Check sheet for the drawn part. Datum: minimum x, y, z corner. Units: mm. Give positions to 0.01 mm unless a question says otherwise; leave off trailing zeros. Order: outer loops, then holes, each group sorted by start corner. A loop starts at its lowest first (then second) coordinate and runs counter-clockwise, first axis right, second up. Notation, with made-up numbers: M -12.75,12.5 L 0.25,12.5 A14 cw 0.25,26.5 Z; hole C 75,23.5 d2. An arc over 180 degrees is marked long. Answer as CSV lines item,"result". Start each with the question number.
Q1. Section check A-A, the plane y = 0.85. Record the boundary of the cut face in (x, z).
Q2. Thickness scan on line 1 (X direction, y = 0.75, z = 48); line 2 (Z direction, x = 23.5, y = 0.65); line 3 (X direction, y = 1.4, z = 7). Record the ranges inside material, lowest first.
Q3. Go/stop test with flat-tipped pins: pin 1 (0.8 mm diameter, centred on y = 1, z = 47, fed in from -X); pin 2 (0.8 mm diameter, centred on y = 1, z = 11.5, fed in from +X); pin 3 (4 mm diameter, centred on x = 17, z = 43.5, fed in from -Y). Record where each tip stops, or that it passes through.
Q4. Section check C-C, the plane x = 12. Record the boundary of the cut face in (y, z) (1 decimal).
Q5. Section check B-B, the plane z = 11.5. Record the boundary of the cut face in (x, y).
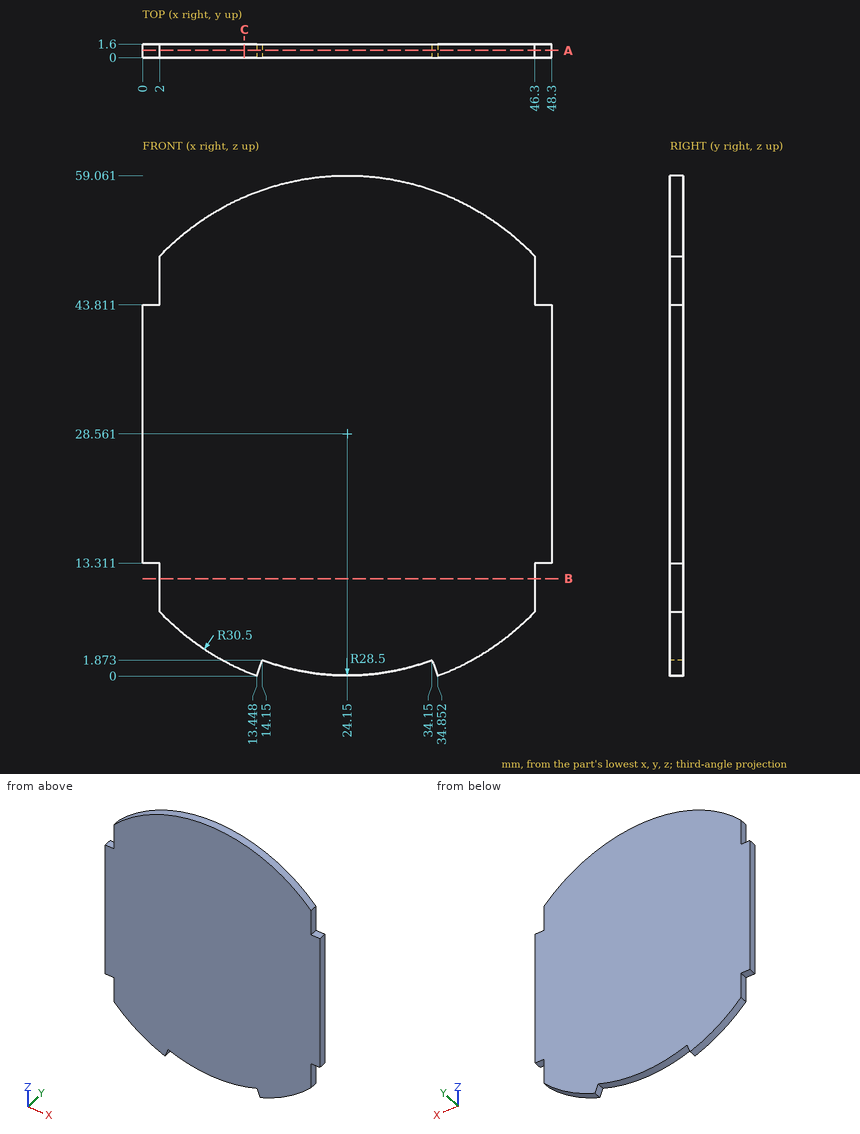
Answer block:
1,outline,"M 0,13.31 L 2,13.31 L 2,7.59 A30.5 ccw 13.45,0 L 14.15,1.87 A28.5 ccw 34.15,1.87 L 34.85,0 A30.5 ccw 46.3,7.59 L 46.3,13.31 L 48.3,13.31 L 48.3,43.81 L 46.3,43.81 L 46.3,49.53 A30.5 ccw 2,49.53 L 2,43.81 L 0,43.81 Z"
2,line 1,"x = 2 to 46.3"
2,line 2,"z = 0.07 to 59.05"
2,line 3,"x = 2.58 to 45.72"
3,pin 1,"stops at x = 2"
3,pin 2,"stops at x = 46.3"
3,pin 3,"stops at y = 0"
4,outline,"M 0,0.6 L 1.6,0.6 L 1.6,56.5 L 0,56.5 Z"
5,outline,"M 2,0 L 46.3,0 L 46.3,1.6 L 2,1.6 Z"
